from build123d import *

# Parameters (mm, degrees)
SKETCH1_R           = 1.5875
BOSS_EXTRUDE1_DEPTH = 5
SKETCH2_W           = 39.37
SKETCH2_H           = 30.4
BOSS_EXTRUDE2_DEPTH = 3.81
SKETCH3_W           = 11.1125
SKETCH3_H           = 10.08
CUT_EXTRUDE1_DEPTH  = 3.81
FILLET1_R           = 2.54
CHAMFER1_SIZE       = 7.62
CHAMFER2_SIZE       = 5.08
BOSS_EXTRUDE3_DEPTH = 2.032
BOSS_EXTRUDE4_DEPTH = 2.032
BOSS_EXTRUDE5_DEPTH = 2.032
BOSS_EXTRUDE6_DEPTH = 2.032
SKETCH8_R           = 1.75
SKETCH8_R_2         = 1.7499965
CUT_EXTRUDE2_DEPTH  = 20.32
SKETCH9_R           = 3
CUT_EXTRUDE3_DEPTH  = 10.16
BOSS_EXTRUDE7_DEPTH = 2.032
BOSS_EXTRUDE8_DEPTH = 2.032


with BuildPart() as part:
    # Sketch1 → Boss-Extrude1 (new body)
    with BuildSketch(Plane(origin=(0, 0, 0), x_dir=(1, 0, 0), z_dir=(0, 1, 0))):
        with BuildLine():
            Line((-33.3375, 0), (-19.685, 0))
            Line((-19.685, 0), (-19.685, 41.68899781))
            Line((-19.685, 41.68899781), (-5.55625, 41.68899781))
            Line((-5.55625, 41.68899781), (-5.55625, 60.73899781))
            Line((-5.55625, 60.73899781), (5.55625, 60.73899781))
            Line((5.55625, 60.73899781), (5.55625, 41.68899781))
            Line((5.55625, 41.68899781), (19.685, 41.68899781))
            Line((19.685, 41.68899781), (19.685, 0))
            Line((19.685, 0), (33.3375, 0))
            Line((33.3375, 0), (33.3375, 85.198868165))
            Line((33.3375, 85.198868165), (9.525, 85.198868165))
            ThreePointArc((9.525, 85.198868165), (0, 75.673868165), (-9.525, 85.198868165))
            Line((-9.525, 85.198868165), (-33.3375, 85.198868165))
            Line((-33.3375, 85.198868165), (-33.3375, 0))
        make_face()
        with Locations(Location((-28.575, 12.975059538, 0), (0, 0, 270))):
            Circle(SKETCH1_R, mode=Mode.SUBTRACT)
        with Locations(Location((28.575, 12.975059538, 0), (0, 0, 270))):
            Circle(SKETCH1_R, mode=Mode.SUBTRACT)
        with Locations(Location((-28.575, 44.725059538, 0), (0, 0, 270))):
            Circle(SKETCH1_R, mode=Mode.SUBTRACT)
        with Locations(Location((-28.575, 78.062559538, 0), (0, 0, 270))):
            Circle(SKETCH1_R, mode=Mode.SUBTRACT)
        with Locations(Location((28.575, 44.725059538, 0), (0, 0, 270))):
            Circle(SKETCH1_R, mode=Mode.SUBTRACT)
        with Locations(Location((28.575, 78.062559538, 0), (0, 0, 270))):
            Circle(SKETCH1_R, mode=Mode.SUBTRACT)
    extrude(amount=BOSS_EXTRUDE1_DEPTH)

    # Sketch2 → Boss-Extrude2 (add)
    with BuildSketch(Plane.XY.offset(-41.68899781)):
        with Locations((0, 2.5)):
            Rectangle(SKETCH2_W, SKETCH2_H)
    extrude(amount=BOSS_EXTRUDE2_DEPTH)

    # Sketch3 → Cut-Extrude1 (cut)
    with BuildSketch(Plane(origin=(0, 0, -41.68899781), x_dir=(-1, 0, 0), z_dir=(0, 0, -1))):
        with Locations((0, 2.5)):
            Rectangle(SKETCH3_W, SKETCH3_H)
    extrude(amount=-CUT_EXTRUDE1_DEPTH, mode=Mode.SUBTRACT)

    # Fillet1
    fillet1_edges = [part.edges().sort_by_distance(p)[0] for p in [
        (5.55625, -2.54, -39.78399781),
        (-5.55625, -2.54, -39.78399781),
        (5.55625, 7.54, -39.78399781),
        (-5.55625, 7.54, -39.78399781),
    ]]
    fillet(fillet1_edges, radius=FILLET1_R)

    # Chamfer1
    chamfer1_edges = [part.edges().sort_by_distance(p)[0] for p in [
        (19.685, -12.7, -39.78399781),
        (-19.685, 17.7, -39.78399781),
        (-19.685, -12.7, -39.78399781),
        (19.685, 17.7, -39.78399781),
    ]]
    chamfer(chamfer1_edges, length=CHAMFER1_SIZE)

    # Chamfer2
    chamfer2_edges = [part.edges().sort_by_distance(p)[0] for p in [
        (19.685, 2.5, 0),
        (-19.685, 2.5, 0),
    ]]
    chamfer(chamfer2_edges, length=CHAMFER2_SIZE)

    # Sketch4 → Boss-Extrude3 (add)
    with BuildSketch(Plane.ZY.offset(-5.55625)):
        Polygon((-41.68899781, 5), (-54.38899781, 5), (-41.68899781, 11.35), align=None)
    extrude(amount=-BOSS_EXTRUDE3_DEPTH)

    # Sketch5 → Boss-Extrude4 (add)
    with BuildSketch(Plane(origin=(-5.55625, 0, 0), x_dir=(0, 0, -1), z_dir=(1, 0, 0))):
        Polygon((54.38899781, 5), (41.68899781, 5), (41.68899781, 11.35), align=None)
    extrude(amount=-BOSS_EXTRUDE4_DEPTH)

    # Sketch6 → Boss-Extrude5 (add)
    with BuildSketch(Plane(origin=(-5.55625, 0, 0), x_dir=(0, 0, -1), z_dir=(1, 0, 0))):
        Polygon((41.68899781, 0), (54.38899781, 0), (41.68899781, -6.35), align=None)
    extrude(amount=-BOSS_EXTRUDE5_DEPTH)

    # Sketch7 → Boss-Extrude6 (add)
    with BuildSketch(Plane.ZY.offset(-5.55625)):
        Polygon((-41.68899781, 0), (-54.38899781, 0), (-41.68899781, -6.35), align=None)
    extrude(amount=-BOSS_EXTRUDE6_DEPTH)

    # Sketch8 → Cut-Extrude2 (cut)
    with BuildSketch(Plane.XY.offset(-37.87899781)):
        with Locations((-8.841749375, 11.716378166)):
            Circle(SKETCH8_R)
        with Locations((8.85825, 11.721080704)):
            Circle(SKETCH8_R)
        with Locations((8.85825, -5.978919296)):
            Circle(SKETCH8_R)
        with Locations((-8.841749375, -5.983621834)):
            Circle(SKETCH8_R_2)
    extrude(amount=-CUT_EXTRUDE2_DEPTH, mode=Mode.SUBTRACT)

    # Sketch9 → Cut-Extrude3 (cut)
    with BuildSketch(Plane(origin=(0, 0, -41.68899781), x_dir=(-1, 0, 0), z_dir=(0, 0, -1))):
        with Locations((-8.85825, 11.721080704)):
            Circle(SKETCH9_R)
        with Locations((8.841749375, 11.716378166)):
            Circle(SKETCH9_R)
        with Locations((8.841749375, -5.983621834)):
            Circle(SKETCH9_R)
        with Locations((-8.85825, -5.978919296)):
            Circle(SKETCH9_R)
    extrude(amount=CUT_EXTRUDE3_DEPTH, mode=Mode.SUBTRACT)

    # Sketch10 → Boss-Extrude7 (add)
    with BuildSketch(Plane(origin=(19.685, 0, 0), x_dir=(0, 0, -1), z_dir=(1, 0, 0))):
        Polygon((41.68899781, 9.971080704), (51.631159218, 5), (41.68899781, 5), align=None)
        Polygon((41.68899781, -5.08), (51.84899781, 0), (41.68899781, 0), align=None)
    extrude(amount=-BOSS_EXTRUDE7_DEPTH)

    # Sketch11 → Boss-Extrude8 (add)
    with BuildSketch(Plane.ZY.offset(19.685)):
        Polygon((-41.68899781, 10.08), (-51.84899781, 5), (-41.68899781, 5), align=None)
        Polygon((-41.68899781, -5.08), (-41.68899781, 0), (-51.84899781, 0), align=None)
    extrude(amount=-BOSS_EXTRUDE8_DEPTH)


solid = part.part
Geometry: final body of the model. Coordinates: model frame, mm. A direction names the side the tool comes from. Round coordinates to 2 decimals unless told otherwise and drop trailing zeros. Loops run counter-clockwise (first coordinate to the right, second up) from the corner with the lowest first, then second, coordinate; pieces in that order, holes last.
Q1. Section B-B on x = 0. Return loops of the section in (y, z), plus the area to 3 significant figures.
Q2. Pull-direction query (X, two-part tool) for faces 1 (the flat face through (-5.556, 3, -47)), 2 (the flat face through (6.332, -2.425, -49.539)), 3 (the flat face through (17.653, -2, -46)), 4 (the flat face through (15.928, 13.837, -39.811)); classes: released by +X, released by -X, zero draft, split by the parting line, or undercut.
Q3. Section A-A on z = -26. Return loops of the section in (x, y) (1 decimal), plus the area to 3 significant figures.
Q4. Access query for faces 5 (the flat face through (19.685, 7, -43)), 6 (the flat face through (22.189, 2.465, -2.576)), 7 (the cylindrical face through (-4.83, 6.78, -39.76)), 8 (the flat face through (-8, 5, -53)), 9 (the flat face through (-8, 0, -53)). Directions: +Z, -Z, +X, -X, +Y, -Y. A direction counts if a zero-diameter tool reaches every point of the face in a straight line with its end or side. Return the directions, or none.
Q5. Material intervals for L1, parallel to X at y = 7, z = -42.5 (3 decimals); L2, parallel to X at y = 4.5, z = -29 (1 decimal); L3, parallel to X at y = 1, z = -53.5, sorted ascending.
Q6. Pin query (flat end, axial travel): P1, Ø4.5, axis at x = 8.86, y = -5.98, coming from the +Z side; P2, Ø6, axis at x = -20, z = -21, coming from the +Y side; P3, Ø2.5, axis at y = 8.5, z = -49, coming from the +X side. Return the tip coordinate at first contact, or that it passes through.
Q7. Section C-C on y = 4. State how many separate pieces and enclosed holes the cut face has, plus the area to 3 significant figures.
Q8. Section D-D on x = 14. Return loops of the section in (y, z) (3 decimals).
Evaluation:
1. outline: (-12.7, -41.69) - (-2.54, -41.69) - (-2.54, -37.88) - (-12.7, -37.88) - close; (0, -75.67) - (5, -75.67) - (5, -60.74) - (0, -60.74) - close; (7.54, -41.69) - (17.7, -41.69) - (17.7, -37.88) - (7.54, -37.88) - close
1. area: 152 mm2
2. face 1: undercut
2. face 2: zero draft
2. face 3: undercut
2. face 4: released by +X
3. outline: (-33.3, 0) - (-19.7, 0) - (-19.7, 5) - (-33.3, 5) - close; (19.7, 0) - (33.3, 0) - (33.3, 5) - (19.7, 5) - close
3. area: 137 mm2
4. face 5: +Z, -Z, +X, +Y
4. face 6: +Z, +Y, -Y
4. face 7: +Z, -Z
4. face 8: -Z, +Y
4. face 9: -Z, -Y
5. L1: x = -19.685 to -17.653, -7.588 to -5.556, 5.556 to 7.588, 17.653 to 19.685
5. L2: x = -33.3 to -19.7, 19.7 to 33.3
5. L3: x = -33.34 to -5.56, 5.56 to 33.34
6. P1: stops at z = -37.88
6. P2: stops at y = 5
6. P3: stops at x = 7.59
7. separate pieces: 1
7. enclosed holes: 6
7. area: 3,720 mm2
8. outline: (-10.765, -41.689) - (0, -41.689) - (0, -85.199) - (5, -85.199) - (5, -41.689) - (15.765, -41.689) - (15.765, -37.879) - (-10.765, -37.879) - close
